Read the model definition and answer for the solid it produces. Units are mm, in the model's axes. A direction names the side the tool comes from. Coordinates: 2 decimals unless noted, no trailing zeros. Write each loop counter-clockwise with the first axis right and the second up, starting at its lowest first coordinate (ties: lowest second). Pieces come first, ordered by that corner, then holes. Notation, with made-up numbers: (-4, 54.25) -> (49, 54.25) arc R28 ccw to (49, 72.25) -> close; hole circle Ø6 at (40.5, 70.25). An arc over 180 degrees is marked (long way). Answer as a JSON object with one key per item and string values. Group by question number.
(1) Find section C-C (x = 5). Give the vertices of the cut face in (y, z), then the cut area to 3 significant figures.
(2) Which of the six approach directions +Z, -Z, +X, -X, +Y, -Y give full straight-line access (tool end or side, diameter ignored) to faces 1 (the face through (5.469, 0, 3)), 2 (the face through (-0.967, 9, 3)), 3 (the face through (4, -1.677, 3))?
(3) Find section D-D (z = 0.8). Count the separate pieces of the cut face and the enclosed holes in it, then the cut area to 3 significant figures.
(4) Find section A-A (y = -1.29). Give the vertices of the cut face in (x, z).
(5) For a pull along Y with two mould halves and no side action, classify faces 4 (the face through (-2, -2.326, 3)), 5 (the face through (-7.26, -8.88, 0.79)), 6 (the face through (-7.105, 0.794, 0.789)), 7 (the face through (-7.78, 0, 1)) as +Y half, -Y half, draft (parallel to the pull), parting line (faces both ways), or undercut.
(6) Flat-ended cylindrical pins translate along their axes: P1, Ø1.6, axis at y = 1, z = 2.5, coming from the +X side; P2, Ø2, axis at x = -6.51, y = 1.25, coming from the +Z side; P3, Ø1, axis at y = 9, z = 2.5, coming from the -X side. Find the tip coordinate at first contact, or state that the pin passes through.
(7) Straight lines are drawn through the part: L1, parallel to Y at x = -2.25, z = 3.4; L2, parallel to X at y = -1, z = 2.5; L3, parallel to Y at x = 4.75, z = 2.65. For each, find the intervals that lie inside material, in ascending order.
(8) Find section B-B (z = 2.6). Give the vertices of the cut face in (x, y).
from build123d import *

# Parameters (mm, degrees)
SKETCH_1_W      = 15.56
SKETCH_1_H      = 20.28
SKETCH_1_R      = 1.5
SKETCH_1_R_2    = 0.75
EXTRUDE_1_DEPTH = 1.6
SKETCH_2_W      = 2.267131812
SKETCH_2_H      = 3.757883692
SKETCH_2_W_2    = 3.109101674
SKETCH_2_H_2    = 4.394457387
SKETCH_2_W_3    = 2.437826046
SKETCH_2_H_3    = 1.976096162
EXTRUDE_2_DEPTH = 2


with BuildPart() as part:
    # 草图1 → 凸台-拉伸1 (new body)
    with BuildSketch(Plane.XY):
        Rectangle(SKETCH_1_W, SKETCH_1_H)
        with Locations((5.24, 7.6)):
            Circle(SKETCH_1_R, mode=Mode.SUBTRACT)
        with Locations((5.24, -7.6)):
            Circle(SKETCH_1_R, mode=Mode.SUBTRACT)
        with Locations((-6.51, 8.87)):
            Circle(SKETCH_1_R_2, mode=Mode.SUBTRACT)
        with Locations((-6.51, 6.33)):
            Circle(SKETCH_1_R_2, mode=Mode.SUBTRACT)
        with Locations((-6.51, 3.79)):
            Circle(SKETCH_1_R_2, mode=Mode.SUBTRACT)
        with Locations((-6.51, 1.25)):
            Circle(SKETCH_1_R_2, mode=Mode.SUBTRACT)
        with Locations((-6.51, -1.29)):
            Circle(SKETCH_1_R_2, mode=Mode.SUBTRACT)
        with Locations((-6.51, -3.83)):
            Circle(SKETCH_1_R_2, mode=Mode.SUBTRACT)
        with Locations((-6.51, -6.37)):
            Circle(SKETCH_1_R_2, mode=Mode.SUBTRACT)
        with Locations((-6.51, -8.91)):
            Circle(SKETCH_1_R_2, mode=Mode.SUBTRACT)
    extrude(amount=EXTRUDE_1_DEPTH)

    # 草图2 → 凸台-拉伸2 (add)
    with BuildSketch(Plane.XY.offset(1.6)):
        with Locations((4.335037476, 0.202355131)):
            Rectangle(SKETCH_2_W, SKETCH_2_H)
        with Locations((-2.143513608, -0.128846081)):
            Rectangle(SKETCH_2_W_2, SKETCH_2_H_2)
        with Locations((-2.18551331, 9.151951919)):
            Rectangle(SKETCH_2_W_3, SKETCH_2_H_3)
    extrude(amount=EXTRUDE_2_DEPTH)


solid = part.part
Results below:
{
 "1": {"outline": "(-10.14, 0) -> (-9.08, 0) -> (-9.08, 1.6) -> (-10.14, 1.6) -> close; (-6.12, 0) -> (6.12, 0) -> (6.12, 1.6) -> (2.08, 1.6) -> (2.08, 3.6) -> (-1.68, 3.6) -> (-1.68, 1.6) -> (-6.12, 1.6) -> close; (9.08, 0) -> (10.14, 0) -> (10.14, 1.6) -> (9.08, 1.6) -> close", "area": "30.5 mm2"},
 "2": {"face 1": "+Z, +X, +Y, -Y", "face 2": "+Z, +X, +Y", "face 3": "+Z, +X, -Y"},
 "3": {"separate pieces": "1", "enclosed holes": "10", "area": "287 mm2"},
 "4": {"outline": "(-7.78, 0) -> (-7.26, 0) -> (-7.26, 1.6) -> (-7.78, 1.6) -> close; (-5.76, 0) -> (7.78, 0) -> (7.78, 1.6) -> (5.47, 1.6) -> (5.47, 3.6) -> (3.2, 3.6) -> (3.2, 1.6) -> (-0.59, 1.6) -> (-0.59, 3.6) -> (-3.7, 3.6) -> (-3.7, 1.6) -> (-5.76, 1.6) -> close"},
 "5": {"face 4": "-Y half", "face 5": "undercut", "face 6": "undercut", "face 7": "draft"},
 "6": {"P1": "stops at x = 5.47", "P2": "stops at z = 1.6", "P3": "stops at x = -3.4"},
 "7": {"L1": "y = -2.33 to 2.07, 8.16 to 10.14", "L2": "x = -3.7 to -0.59, 3.2 to 5.47", "L3": "y = -1.68 to 2.08"},
 "8": {"outline": "(-3.7, -2.33) -> (-0.59, -2.33) -> (-0.59, 2.07) -> (-3.7, 2.07) -> close; (-3.4, 8.16) -> (-0.97, 8.16) -> (-0.97, 10.14) -> (-3.4, 10.14) -> close; (3.2, -1.68) -> (5.47, -1.68) -> (5.47, 2.08) -> (3.2, 2.08) -> close"}
}
